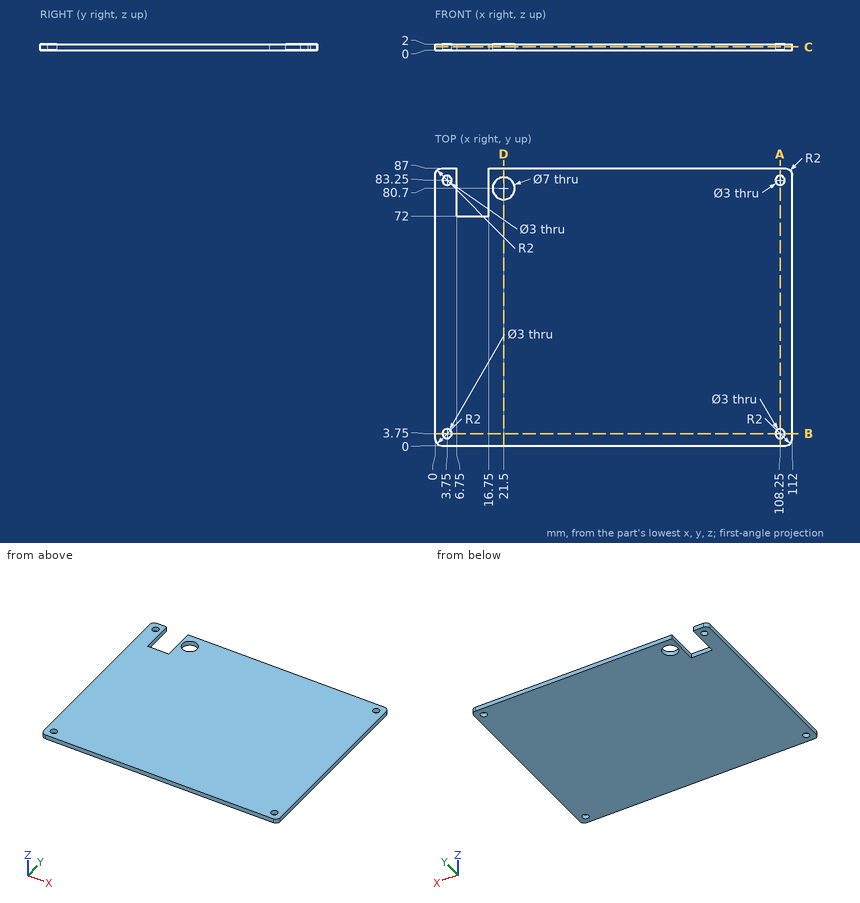
The drawing under review shows one solid part. Ordinate dimensions are in mm from its lowest x, y, z. Coordinates: 2 decimals unless noted, no trailing zeros. Order: outer loops, then holes, each group sorted by start corner. A loop starts at its lowest first (then second) coordinate and runs counter-clockwise, first axis right, second up. Notation, with made-up numbers: (45, 67.5) -> (80, 67.5) arc R13 cw to (80, 81.5) -> close; hole circle Ø1 at (35.5, 10.5). An arc over 180 degrees is marked (long way). Answer as CSV lines item,"result".
Q1. We need section A-A (x = 108.25). State the section outline as (y, z) points.
Model answer:
outline,"(0, 0) -> (2.25, 0) -> (2.25, 2) -> (0, 2) -> close; (5.25, 0) -> (81.75, 0) -> (81.75, 2) -> (5.25, 2) -> close; (84.75, 0) -> (87, 0) -> (87, 2) -> (84.75, 2) -> close"
Q2. We need section B-B (y = 3.75). State the section outline as (x, z) points, plus the area to 3 significant figures.
Model answer:
outline,"(0, 0) -> (2.25, 0) -> (2.25, 2) -> (0, 2) -> close; (5.25, 0) -> (106.75, 0) -> (106.75, 2) -> (5.25, 2) -> close; (109.75, 0) -> (112, 0) -> (112, 2) -> (109.75, 2) -> close"
area,"212 mm2"
Q3. Wall thickness on line 1 along Y through (x, z) = (108.25, 1.05); line 2 along Y through (x, z) = (24.5, 0.1); line 3 along Y through (x, z) = (15.5, 0.9): over which ranges is each line inside the solid? List them lowest first. Write a range as [from, to].
Model answer:
line 1,"y = [0, 2.25], [5.25, 81.75], [84.75, 87]"
line 2,"y = [0, 78.9], [82.5, 87]"
line 3,"y = [0, 72]"
Q4. We need section C-C (z = 1.1). State the section outline as (x, y) points.
Model answer:
outline,"(0, 2) arc R2 ccw to (2, 0) -> (110, 0) arc R2 ccw to (112, 2) -> (112, 85) arc R2 ccw to (110, 87) -> (16.75, 87) -> (16.75, 72) -> (6.75, 72) -> (6.75, 87) -> (2, 87) arc R2 ccw to (0, 85) -> close; hole circle Ø3 at (3.75, 3.75); hole circle Ø3 at (3.75, 83.25); hole circle Ø7 at (21.5, 80.7); hole circle Ø3 at (108.25, 3.75); hole circle Ø3 at (108.25, 83.25)"
Q5. Clearance check with flat-ended pins moving along their axes: pin 1 Ø1 at (y, z) = (34, 1.5) entering from -X; pin 2 Ø2.5 at (x, y) = (108.25, 83.25) entering from -Z. State where each tip first meets the part, or that it passes through.
Model answer:
pin 1,"stops at x = 0"
pin 2,"passes through"
Q6. We need section D-D (x = 21.5). State the section outline as (y, z) points.
Model answer:
outline,"(0, 0) -> (77.2, 0) -> (77.2, 2) -> (0, 2) -> close; (84.2, 0) -> (87, 0) -> (87, 2) -> (84.2, 2) -> close"
